For this review, take the finished solid that the model builds, in its own axes (mm). Round coordinates to 2 decimals unless told otherwise and drop trailing zeros. Write each loop counter-clockwise with the first axis right and the second up, starting at its lowest first coordinate (ties: lowest second). Pieces come first, ordered by that corner, then holes. Notation, with made-up numbers: M -38,6 L -14,6 A10 ccw -14,19 Z; hole C 40.25,-20.75 d9. An arc over 180 degrees is marked long. One line per question, with ' | ' between items.
```python
from build123d import *

# Parameters (mm, degrees)
F0_R     = 31.75
F1_DEPTH = 25.4


with BuildPart() as f1:
    # F0 (on Front) → F1 (new body)
    with BuildSketch(Plane.XZ):
        Circle(F0_R)
        with BuildLine():
            ThreePointArc((18.7028452874, 12.0064234124), (20.5332226101, 8.5051392843), (21.7147321429, 4.7350853175))
            ThreePointArc((21.7147321429, 4.7350853175), (25.4070791615, 3.543413391), (26.9875, 0))
            ThreePointArc((26.9875, 0), (25.4070791615, -3.543413391), (21.7147321429, -4.7350853175))
            ThreePointArc((21.7147321429, -4.7350853175), (20.5332226101, -8.5051392843), (18.7028452874, -12.0064234124))
            ThreePointArc((18.7028452874, -12.0064234124), (20.0113116188, -13.6594900802), (20.4779482119, -15.7154482119))
            ThreePointArc((20.4779482119, -15.7154482119), (17.2993004213, -20.2068642947), (12.0064234124, -18.7028452874))
            ThreePointArc((12.0064234124, -18.7028452874), (8.5051392843, -20.5332226101), (4.7350853175, -21.7147321429))
            ThreePointArc((4.7350853175, -21.7147321429), (4.7556413907, -21.969498116), (4.7625, -22.225))
            ThreePointArc((4.7625, -22.225), (-0.255501884, -26.9806413907), (-4.7350853175, -21.7147321429))
            ThreePointArc((-4.7350853175, -21.7147321429), (-8.5051392843, -20.5332226101), (-12.0064234124, -18.7028452874))
            ThreePointArc((-12.0064234124, -18.7028452874), (-19.0830442573, -19.0830442573), (-18.7028452874, -12.0064234124))
            ThreePointArc((-18.7028452874, -12.0064234124), (-20.5332226101, -8.5051392843), (-21.7147321429, -4.7350853175))
            ThreePointArc((-21.7147321429, -4.7350853175), (-26.9875, 0), (-21.7147321429, 4.7350853175))
            ThreePointArc((-21.7147321429, 4.7350853175), (-20.5332226101, 8.5051392843), (-18.7028452874, 12.0064234124))
            ThreePointArc((-18.7028452874, 12.0064234124), (-19.0830442573, 19.0830442573), (-12.0064234124, 18.7028452874))
            ThreePointArc((-12.0064234124, 18.7028452874), (-8.5051392843, 20.5332226101), (-4.7350853175, 21.7147321429))
            ThreePointArc((-4.7350853175, 21.7147321429), (-0.255501884, 26.9806413907), (4.7625, 22.225))
            ThreePointArc((4.7625, 22.225), (4.7556413907, 21.969498116), (4.7350853175, 21.7147321429))
            ThreePointArc((4.7350853175, 21.7147321429), (8.5051392843, 20.5332226101), (12.0064234124, 18.7028452874))
            ThreePointArc((12.0064234124, 18.7028452874), (17.2993004213, 20.2068642947), (20.4779482119, 15.7154482119))
            ThreePointArc((20.4779482119, 15.7154482119), (20.0113116188, 13.6594900802), (18.7028452874, 12.0064234124))
        make_face(mode=Mode.SUBTRACT)
        with BuildLine():
            ThreePointArc((21.7147321429, -4.7350853175), (17.4625, 0), (21.7147321429, 4.7350853175))
            ThreePointArc((21.7147321429, 4.7350853175), (20.5332226101, 8.5051392843), (18.7028452874, 12.0064234124))
            ThreePointArc((18.7028452874, 12.0064234124), (12.3478521665, 12.3478521665), (12.0064234124, 18.7028452874))
            ThreePointArc((12.0064234124, 18.7028452874), (8.5051392843, 20.5332226101), (4.7350853175, 21.7147321429))
            ThreePointArc((4.7350853175, 21.7147321429), (0, 17.4625), (-4.7350853175, 21.7147321429))
            ThreePointArc((-4.7350853175, 21.7147321429), (-8.5051392843, 20.5332226101), (-12.0064234124, 18.7028452874))
            ThreePointArc((-12.0064234124, 18.7028452874), (-11.2240321291, 17.2993004213), (-10.9529482119, 15.7154482119))
            ThreePointArc((-10.9529482119, 15.7154482119), (-13.6594900802, 11.4195848049), (-18.7028452874, 12.0064234124))
            ThreePointArc((-18.7028452874, 12.0064234124), (-20.5332226101, 8.5051392843), (-21.7147321429, 4.7350853175))
            ThreePointArc((-21.7147321429, 4.7350853175), (-18.681586609, 3.1820791615), (-17.4625, 0))
            ThreePointArc((-17.4625, 0), (-18.681586609, -3.1820791615), (-21.7147321429, -4.7350853175))
            ThreePointArc((-21.7147321429, -4.7350853175), (-20.5332226101, -8.5051392843), (-18.7028452874, -12.0064234124))
            ThreePointArc((-18.7028452874, -12.0064234124), (-13.6594900802, -11.4195848049), (-10.9529482119, -15.7154482119))
            ThreePointArc((-10.9529482119, -15.7154482119), (-11.2240321291, -17.2993004213), (-12.0064234124, -18.7028452874))
            ThreePointArc((-12.0064234124, -18.7028452874), (-8.5051392843, -20.5332226101), (-4.7350853175, -21.7147321429))
            ThreePointArc((-4.7350853175, -21.7147321429), (0, -17.4625), (4.7350853175, -21.7147321429))
            ThreePointArc((4.7350853175, -21.7147321429), (8.5051392843, -20.5332226101), (12.0064234124, -18.7028452874))
            ThreePointArc((12.0064234124, -18.7028452874), (12.3478521665, -12.3478521665), (18.7028452874, -12.0064234124))
            ThreePointArc((18.7028452874, -12.0064234124), (20.5332226101, -8.5051392843), (21.7147321429, -4.7350853175))
        make_face()
    extrude(amount=F1_DEPTH)


solid = f1.part
```
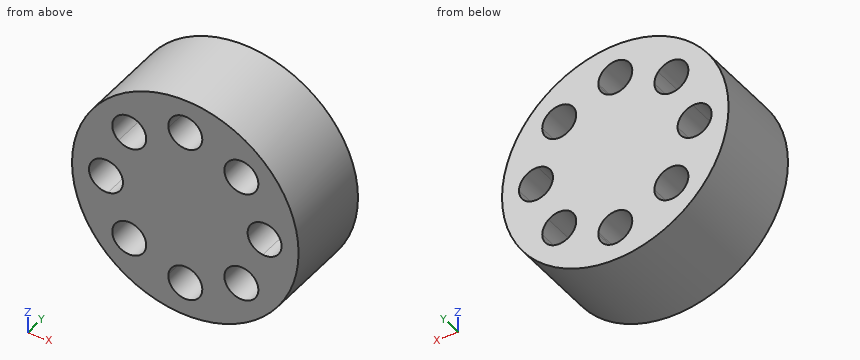
Item 1: To check wall thickness, follow line 1 along Z through (x, y) = (-0.5, -11.75); line 2 along Z through (x, y) = (2, -18.75); line 3 along X through (y, z) = (-23.5, -13.5). State the ranges of each line that lie inside material, in increasing order. Write a range as from..to.
Results:
line 1: -31.75..-26.96, -17.49..17.49, 26.96..31.75 | line 2: -31.69..-26.55, -17.9..17.9, 26.55..31.69 | line 3: -28.74..-19.93, -11.5..11.5, 19.93..28.74
Item 2: Take a section at A-A (x = 0). Write out the cut boundary in (y, z).
Results:
outline: M -25.4,-31.75 L 0,-31.75 L 0,-26.99 L -25.4,-26.99 Z; M -25.4,-17.46 L 0,-17.46 L 0,17.46 L -25.4,17.46 Z; M -25.4,26.99 L 0,26.99 L 0,31.75 L -25.4,31.75 Z
Item 3: Take a section at C-C (x = 14). Write out the cut boundary in (y, z).
Results:
outline: M -25.4,-28.5 L 0,-28.5 L 0,-20.16 L -25.4,-20.16 Z; M -25.4,-11.27 L 0,-11.27 L 0,11.27 L -25.4,11.27 Z; M -25.4,20.16 L 0,20.16 L 0,28.5 L -25.4,28.5 Z
Item 4: Insertion check: pin 1 Ø10 at (x, y) = (7.5, -5.5) entering from +Z; pin 2 Ø6 at (x, y) = (-7, -20) entering from -Z; pin 3 Ø4 at (x, y) = (-9.5, -12.5) entering from +Z. Each pin has a flat end and moves straight along its axis. Give the tip position at first contact, or say it passes through.
Results:
pin 1: z = 31.65 | pin 2: z = -31.5 | pin 3: z = 30.85
Item 5: Take a section at D-D (z = -10). Write out the cut boundary in (x, y).
Results:
outline: M -30.13,-25.4 L 30.13,-25.4 L 30.13,0 L -30.13,0 Z
Item 6: Take a section at B-B (y = -8.25). State how many separate pieces and enclosed holes the cut face has, then the cut area to 3 significant figures.
Results:
separate pieces: 1 | enclosed holes: 8 | area: 2,600 mm2
